Verification items for the finished model (mm, model axes). Round coordinates to 2 decimals unless told otherwise and drop trailing zeros. Write each loop counter-clockwise with the first axis right and the second up, starting at its lowest first coordinate (ties: lowest second). Pieces come first, ordered by that corner, then holes.
from build123d import *

# Parameters (mm, degrees)
SKETCH1_R            = 2.0828
BOSS_EXTRUDE1_DEPTH  = 3.175
M3_CLEARANCE_HOLE1_D = 3.2


with BuildPart() as part:
    # Sketch1 → Boss-Extrude1 (new body)
    with BuildSketch(Plane(origin=(0, 0, 0), x_dir=(1, 0, 0), z_dir=(0, 1, 0))):
        Polygon((28.855389821, 184.15), (123.544610179, 184.15), (176.5, 131.194610179), (176.5, 111.76), (182.5, 111.76), (182.5, 125.194610179), (190.5, 117.194610179), (190.5, 22.505389821), (182.5, 14.505389821), (182.5, 27.94), (176.5, 27.94), (176.5, 8.505389821), (137.544610179, -30.45), (118.11, -30.45), (118.11, -36.45), (131.544610179, -36.45), (123.544610179, -44.45), (28.855389821, -44.45), (20.855389821, -36.45), (34.29, -36.45), (34.29, -30.45), (14.855389821, -30.45), (-24.1, 8.505389821), (-24.1, 27.94), (-30.1, 27.94), (-30.1, 14.505389821), (-38.1, 22.505389821), (-38.1, 117.194610179), (-30.1, 125.194610179), (-30.1, 111.76), (-24.1, 111.76), (-24.1, 131.194610179), align=None)
        with Locations(Location((24.384, 12.7, 0), (0, 0, 270))):
            Circle(SKETCH1_R, mode=Mode.SUBTRACT)
        with Locations(Location((128.016, 12.7, 0), (0, 0, 90))):
            Circle(SKETCH1_R, mode=Mode.SUBTRACT)
        with Locations(Location((128.016, 127, 0), (0, 0, 270))):
            Circle(SKETCH1_R, mode=Mode.SUBTRACT)
        with Locations(Location((24.384, 127, 0), (0, 0, 90))):
            Circle(SKETCH1_R, mode=Mode.SUBTRACT)
    extrude(amount=BOSS_EXTRUDE1_DEPTH)

    # M3 Clearance Hole1 (through all)
    with Locations(Plane(origin=(0, 3.175, 0), x_dir=(1, 0, 0), z_dir=(0, 1, 0))):
        with Locations((-19.05, 127), (-19.05, 111.76), (-19.05, 27.94), (-19.05, 12.7), (171.45, 127), (171.45, 111.76), (171.45, 27.94), (171.45, 12.7), (133.35, -25.4), (118.11, -25.4), (34.29, -25.4), (19.05, -25.4)):
            Hole(M3_CLEARANCE_HOLE1_D / 2)


solid = part.part
Q1. Sectioned sample at B-B (x = 0). Enter the section's corners in (y, z) (3 decimals).
Recorded:
outline: (0, -155.295) - (3.175, -155.295) - (3.175, 15.595) - (0, 15.595) - close
Q2. Material ranges on line 1 along X through (y, z) = (2.2, -13); line 2 along Z through (x, y) = (-19.05, 2.15); line 3 along X through (y, z) = (2, 25.4), recorded low to high.
Recorded:
line 1: x = -24.1 to -20.62, -17.48 to 22.32, 26.45 to 125.95, 130.08 to 169.88, 173.02 to 176.5
line 2: z = -136.24 to -128.6, -125.4 to -113.36, -110.16 to -29.54, -26.34 to -14.3, -11.1 to -3.46
line 3: x = 9.81 to 17.45, 20.65 to 32.69, 35.89 to 116.51, 119.71 to 131.75, 134.95 to 142.59
Q3. Sectioned sample at A-A (y = 2.65). Give the number of separate pieces and of enclosed holes in the cut face, plus the area to 3 significant figures.
Recorded:
separate pieces: 1
enclosed holes: 16
area: 42,500 mm2
Q4. Sectioned sample at C-C (z = -166). Enter the section's corners in (x, y) (3 decimals), plus the area to 3 significant figures.
Recorded:
outline: (10.705, 0) - (141.695, 0) - (141.695, 3.175) - (10.705, 3.175) - close
area: 416 mm2
Q5. Depth check by flat-ended pin: P1, Ø1, axis at x = -28.5, y = 1.5, coming from the +Z side; P2, Ø2.5, axis at x = -19.05, z = -27.94, coming from the -Y side; P3, Ø1.6, axis at y = 1.5, z = -125.5, coming from the -X side. Enter the tip coordinate at first touch or a pass-through.
Recorded:
P1: stops at z = -27.94
P2: passes through
P3: stops at x = -30.59
